Source: CAD feature listing. Evaluate the final solid. Frame: model axes, mm. Round coordinates to 2 decimals unless told otherwise and drop trailing zeros. Loops run counter-clockwise (first coordinate to the right, second up) from the corner with the lowest first, then second, coordinate; pieces in that order, holes last. Notation, with made-up numbers: M -16.75,26.5 L 2.25,26.5 A31 ccw 2.25,50.5 Z; hole C 64.25,29 d11. An arc over 180 degrees is marked long. Answer as a JSON object with one key per item and string values.
from build123d import *

# Parameters (mm, degrees)
SKETCH_1_R      = 60
SKETCH_1_R_2    = 1.25
SKETCH_1_R_3    = 1
EXTRUDE_1_DEPTH = 3


with BuildPart() as part:
    # 草图1 → 凸台-拉伸1 (new body)
    with BuildSketch(Plane.XY):
        Circle(SKETCH_1_R)
        with Locations((55, 0)):
            Circle(SKETCH_1_R_2, mode=Mode.SUBTRACT)
        with Locations((0, 55)):
            Circle(SKETCH_1_R_2, mode=Mode.SUBTRACT)
        with Locations((0, -55)):
            Circle(SKETCH_1_R_2, mode=Mode.SUBTRACT)
        with Locations((-55, 0)):
            Circle(SKETCH_1_R_2, mode=Mode.SUBTRACT)
        with Locations((0, 20)):
            Circle(SKETCH_1_R_3, mode=Mode.SUBTRACT)
        with Locations((17.320508076, -10)):
            Circle(SKETCH_1_R_3, mode=Mode.SUBTRACT)
        with Locations((-17.320508076, -10)):
            Circle(SKETCH_1_R_3, mode=Mode.SUBTRACT)
        Polygon((35.991735162, 17.606958852), (30.334880913, 23.263813101), (32.456201256, 25.385133445), (38.113055506, 19.728279195), align=None, mode=Mode.SUBTRACT)
        Polygon((23.263813101, 30.334880913), (25.385133445, 32.456201256), (19.728279195, 38.113055506), (17.606958852, 35.991735162), align=None, mode=Mode.SUBTRACT)
        Polygon((11.950104602, 37.405948725), (14.071424946, 35.284628381), (8.414570696, 29.627774132), (6.293250353, 31.749094475), align=None, mode=Mode.SUBTRACT)
        Polygon((31.749094475, 6.293250353), (37.405948725, 11.950104602), (35.284628381, 14.071424946), (29.627774132, 8.414570696), align=None, mode=Mode.SUBTRACT)
        Polygon((29.981327522, 32.102647866), (32.102647866, 29.981327522), (37.759502115, 35.638181772), (35.638181772, 37.759502115), align=None, mode=Mode.SUBTRACT)
    extrude(amount=EXTRUDE_1_DEPTH)


solid = part.part
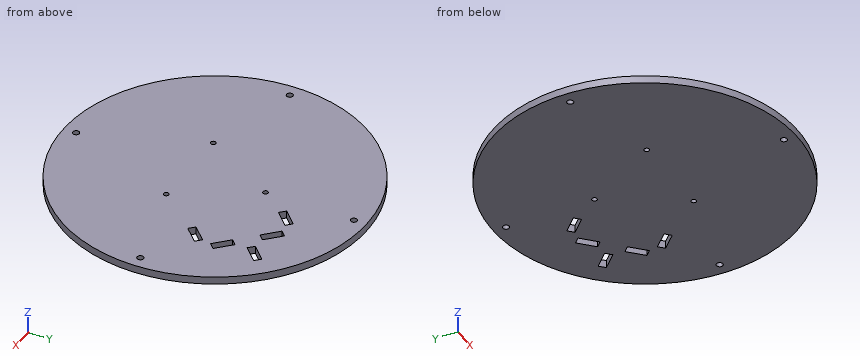
Item 1: Contact query for flat-ended pins moving along their axis: pin 1 Ø1.5 at (y, z) = (20, 1.5) entering from +X; pin 2 Ø1 at (x, z) = (-33.5, 1.5) entering from +Y; pin 3 Ø1 at (x, z) = (18, 2.5) entering from -Y. Output: stop coordinate, or through.
Answer sheet:
{"pin 1": "stops at x = 56.83", "pin 2": "stops at y = 50.11", "pin 3": "stops at y = -57.39"}
Item 2: Line query: probe 1 along Y at (x, z) = (0, 1.2); probe 2 along Y at (x, z) = (31, 2.05); probe 3 along Y at (x, z) = (-17.5, 1.3). Output: solid intervals per line, ascending. Write a range as from..to.
Answer sheet:
{"probe 1": "y = -60..-56.25, -53.75..19, 21..53.75, 56.25..60", "probe 2": "y = -51.37..7.04, 9.79..22.6, 23.93..31.08, 33.12..51.37", "probe 3": "y = -57.39..-10.98, -9.02..57.39"}
Item 3: Section B-B on x = 10.5. Return the cut outline in (y, z), then the cut area to 3 significant figures.
Answer sheet:
{"outline": "M -59.07,0 L 31.71,0 L 31.71,3 L -59.07,3 Z; M 35.96,0 L 59.07,0 L 59.07,3 L 35.96,3 Z", "area": "342 mm²"}
Item 4: Section A-A on z = 1.75. Give the number of separate pieces and of enclosed holes in the cut face, then the cut area to 3 significant figures.
Answer sheet:
{"separate pieces": "1", "enclosed holes": "12", "area": "11,200 mm²"}
Item 5: Section D-D on x = -43. Return the cut outline in (y, z), then the cut area to 3 significant figures.
Answer sheet:
{"outline": "M -41.84,0 L 41.84,0 L 41.84,3 L -41.84,3 Z", "area": "251 mm²"}
Item 6: Section C-C on y = 46. Return the cut outline in (x, z).
Answer sheet:
{"outline": "M -38.52,0 L 38.52,0 L 38.52,3 L -38.52,3 Z"}
